```python
from build123d import *

# Parameters (mm, degrees)
BOX_W             = 80
BOX_H             = 20
BOX_DEPTH         = 2.5
CYLINDER_R        = 4
CYLINDER_DEPTH    = 38
CYLINDER001_R     = 2
CYLINDER001_DEPTH = 38
CYLINDER002_R     = 2.25
CYLINDER002_DEPTH = 2.5
CYLINDER003_R     = 2.25
CYLINDER003_DEPTH = 2.5


with BuildPart() as part:
    # Box → Box (join)
    with BuildSketch(Plane.XY):
        with Locations((40, 10)):
            Rectangle(BOX_W, BOX_H)
    extrude(amount=BOX_DEPTH)

    # Cylinder → Cylinder (join)
    with BuildSketch(Plane(origin=(42, 4, 6), x_dir=(0, 1, 0), z_dir=(1, 0, 0))):
        Circle(CYLINDER_R)
    extrude(amount=CYLINDER_DEPTH)

    # Cylinder001 → Cylinder001 (cut)
    with BuildSketch(Plane(origin=(42, 4, 6), x_dir=(0, 1, 0), z_dir=(1, 0, 0))):
        Circle(CYLINDER001_R)
    extrude(amount=CYLINDER001_DEPTH, mode=Mode.SUBTRACT)

    # Cylinder002 → Cylinder002 (cut)
    with BuildSketch(Plane(origin=(8, 14, 0), x_dir=(0, -1, 0), z_dir=(0, 0, 1))):
        Circle(CYLINDER002_R)
    extrude(amount=CYLINDER002_DEPTH, mode=Mode.SUBTRACT)

    # Cylinder003 → Cylinder003 (cut)
    with BuildSketch(Plane(origin=(74, 14, 0), x_dir=(1, 0, 0), z_dir=(0, 0, 1))):
        Circle(CYLINDER003_R)
    extrude(amount=CYLINDER003_DEPTH, mode=Mode.SUBTRACT)


solid = part.part
```
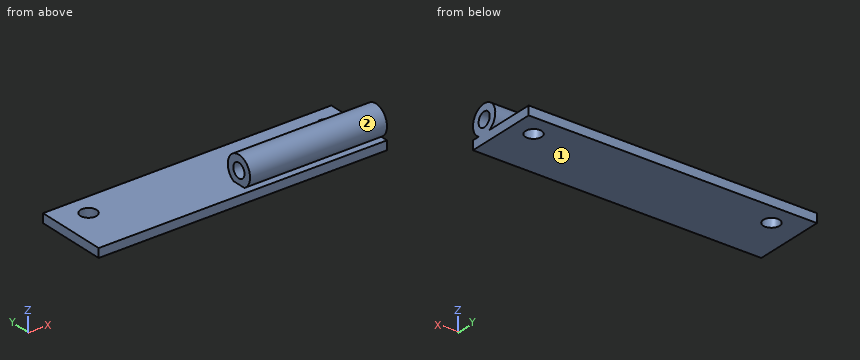
Can you work these out from the model? Positions are in its coordinate system, mm. Face numbers are marked on the shaded views. Coordinates: 2 decimals unless noted, no trailing zeros. Write each loop counter-clockwise with the first axis right and the second up, starting at its lowest first coordinate (ties: lowest second). Pieces come first, ordered by that corner, then holes. Notation, with made-up numbers: M -31,-33.5 L -2,-33.5 A9 ccw -2,-22.5 Z; hole C -23.5,-39.75 d11. An arc over 180 degrees is marked long. Answer as CSV lines item,"result".
Item 1: Imagine slicing it at A-A on x = 8. List the corners of the cut face in (y, z) for me.
Geometry results:
outline,"M 0,0 L 11.75,0 L 11.75,2.5 L 0,2.5 Z; M 16.25,0 L 20,0 L 20,2.5 L 16.25,2.5 Z"
Item 2: I'm going to push flat-ended pins straight in: P1, Ø5, axis at x = 8, y = 14, coming from the +Z side; P2, Ø3.5, axis at x = 74, y = 14, coming from the -Z side; P3, Ø5, axis at x = 64.5, z = 8.5, coming from the +Y side. Where does each tip first touch, or does it pass through?
Geometry results:
P1,"stops at z = 2.5"
P2,"passes through"
P3,"stops at y = 8"
Item 3: We'd pull the mould along Z, two halves only. Please class the marked faces 1 and 2: +Z half, -Z half, draft (parallel to the pull), parting line (faces both ways), or undercut.
Geometry results:
face 1,"-Z half"
face 2,"undercut"
Item 4: Imagine slicing it at C-C on y = 14. List the corners of the cut face in (x, z) for me.
Geometry results:
outline,"M 0,0 L 5.75,0 L 5.75,2.5 L 0,2.5 Z; M 10.25,0 L 71.75,0 L 71.75,2.5 L 10.25,2.5 Z; M 76.25,0 L 80,0 L 80,2.5 L 76.25,2.5 Z"
Item 5: Imagine slicing it at D-D on y = 4. List the corners of the cut face in (x, z) for me, plus the area to 3 significant figures.
Geometry results:
outline,"M 0,0 L 80,0 L 80,4 L 42,4 L 42,2.5 L 0,2.5 Z; M 42,8 L 80,8 L 80,10 L 42,10 Z"
area,"333 mm2"
Item 6: Imagine slicing it at B-B on z = 6. List the corners of the cut face in (x, y) for me, plus the area to 3 significant figures.
Geometry results:
outline,"M 42,0 L 80,0 L 80,2 L 42,2 Z; M 42,6 L 80,6 L 80,8 L 42,8 Z"
area,"152 mm2"
Item 7: Please list where these lines run through material, in increasing order: line 1 along Y through (x, z) = (74, 1.95); line 2 along Z through (x, y) = (54, 4); line 3 along Z through (x, y) = (47.5, 14.5).
Geometry results:
line 1,"y = 0 to 11.75, 16.25 to 20"
line 2,"z = 0 to 4, 8 to 10"
line 3,"z = 0 to 2.5"
